```python
from build123d import *

# Parameters (mm, degrees)
F1_DEPTH = 3.175
F2_R     = 2.38125
F3_DEPTH = 3.175
F4_R     = 7.62
F4_R_2   = 2.032
F5_DEPTH = 25.4


# Not quite as in the source:
# - a feature names something its author has since deleted; it is built from what else it names


with BuildPart() as f1:
    # F0 (on Top) → F1 (new body)
    with BuildSketch(Plane.XY):
        with BuildLine():
            Line((12.7, 0), (12.7, 47.3970452561))
            ThreePointArc((12.7, 47.3970452561), (0, 50.8), (-12.7, 47.3970452561))
            Line((-12.7, 47.3970452561), (-12.7, 0))
            Line((-12.7, 0), (0, 0))
            Line((0, 0), (12.7, 0))
        make_face()
        with BuildLine():
            Line((12.7, -47.3970452561), (12.7, 0))
            Line((12.7, 0), (0, 0))
            Line((0, 0), (-12.7, 0))
            Line((-12.7, 0), (-12.7, -47.3970452561))
            ThreePointArc((-12.7, -47.3970452561), (0, -50.8), (12.7, -47.3970452561))
        make_face()
    extrude(amount=F1_DEPTH)

    # F2 (on face) → F3 (cut, through all)
    with BuildSketch(Plane.XY.offset(3.175)):
        with Locations((-7.9375, 41.275)):
            Circle(F2_R)
        with Locations((7.9375, 41.275)):
            Circle(F2_R)
        with Locations((-7.9375, -34.925)):
            Circle(F2_R)
        with Locations((7.9375, -34.925)):
            Circle(F2_R)
    extrude(amount=-F3_DEPTH, mode=Mode.SUBTRACT)

    # F4 (on face) → F5 (cut)
    with BuildSketch(Plane.XY.offset(3.175)):
        with Locations((0, 19.05)):
            Circle(F4_R)
        with BuildLine():
            ThreePointArc((-11.0199479175, 19.05), (-10.16, 20.955), (-11.0199479175, 22.86))
            ThreePointArc((-11.0199479175, 22.86), (-10.3240475594, 25.6630256121), (-12.7, 27.305))
            Line((-12.7, 27.305), (-12.7, 23.495))
            Line((-12.7, 23.495), (-12.7, 22.225))
            Line((-12.7, 22.225), (-12.7, 19.685))
            Line((-12.7, 19.685), (-12.7, 18.415))
            Line((-12.7, 18.415), (-12.7, 15.875))
            Line((-12.7, 15.875), (-12.7, 14.605))
            Line((-12.7, 14.605), (-12.7, 10.795))
            ThreePointArc((-12.7, 10.795), (-10.3240475594, 12.4369743879), (-11.0199479175, 15.24))
            ThreePointArc((-11.0199479175, 15.24), (-10.16, 17.145), (-11.0199479175, 19.05))
        make_face()
        with BuildLine():
            Line((12.7, 10.795), (12.7, 27.305))
            ThreePointArc((12.7, 27.305), (10.3240475594, 25.6630256121), (11.0199479175, 22.86))
            ThreePointArc((11.0199479175, 22.86), (10.16, 20.955), (11.0199479175, 19.05))
            ThreePointArc((11.0199479175, 19.05), (10.16, 17.145), (11.0199479175, 15.24))
            ThreePointArc((11.0199479175, 15.24), (10.3240475594, 12.4369743879), (12.7, 10.795))
        make_face()
        with Locations((0, 44.45)):
            Circle(F4_R_2)
    extrude(amount=-F5_DEPTH, mode=Mode.SUBTRACT)


solid = f1.part
```
CAD build for the part. Positions are in the model's coordinates, mm. Round coordinates to 2 decimals unless told otherwise and drop trailing zeros. Order: outer loops, then holes, each group sorted by start corner. A loop starts at its lowest first (then second) coordinate and runs counter-clockwise, first axis right, second up. Notation, with made-up numbers: (56.25, 27) -> (78.25, 27) arc R20 cw to (78.25, 34) -> close; hole circle Ø1 at (86, 53.25). An arc over 180 degrees is marked (long way). One line per question, with ' | ' between items.
Q1. Drop a flat-ended pin along its axis: pin 1 (4 mm diameter, centred on x = -7.94, y = 41.28, fed in from -Z). Give the stop position or say it passes through.
Completed:
pin 1: passes through
Q2. Slice it at C-C (z = 1.6). Give the number of separate pieces and of enclosed holes in the cut face, then the cut area to 3 significant figures.
Completed:
separate pieces: 1 | enclosed holes: 6 | area: 2,190 mm^2
Q3. Probe probe 1 along Y at (x, z) = (0, 0.7); probe 2 along Y at (x, z) = (7, 2.15); probe 3 along Y at (x, z) = (1, 3.05). List the from-to ranges inside material, lowest first.
Completed:
probe 1: y = -50.8 to 11.43, 26.67 to 42.42, 46.48 to 50.8 | probe 2: y = -49.82 to -37.11, -32.74 to 16.04, 22.06 to 39.09, 43.46 to 49.82 | probe 3: y = -50.78 to 11.5, 26.6 to 42.68, 46.22 to 50.78
Q4. Slice it at B-B (x = 4.5). Write the cut outline in (y, z) (3 decimals), then the cut area to 3 significant figures.
Completed:
outline: (-50.398, 0) -> (12.901, 0) -> (12.901, 3.175) -> (-50.398, 3.175) -> close; (25.199, 0) -> (50.398, 0) -> (50.398, 3.175) -> (25.199, 3.175) -> close | area: 281 mm^2
Q5. Slice it at A-A (x = 0.5). Write the cut outline in (y, z) (3 decimals).
Completed:
outline: (-50.795, 0) -> (11.446, 0) -> (11.446, 3.175) -> (-50.795, 3.175) -> close; (26.654, 0) -> (42.48, 0) -> (42.48, 3.175) -> (26.654, 3.175) -> close; (46.42, 0) -> (50.795, 0) -> (50.795, 3.175) -> (46.42, 3.175) -> close
Q6. Two-plate mould, pull along X, no slides. Class faces 1 (the cylindrical face through (10.16, 20.99, 1.61)), 2 (the cylindrical face through (5.56, 41.38, 1.61)), 3 (the flat face through (-12.7, 37, 2)): released by +X, released by -X, zero draft, split by the parting line, or undercut.
Completed:
face 1: released by +X | face 2: undercut | face 3: released by -X
